from build123d import *

# Parameters (mm, degrees)
BOSS_EXTRUDE1_DEPTH = 5
SKETCH3_R           = 2.125
CUT_EXTRUDE1_DEPTH  = 10
FILLET1_R           = 10
SKETCH4_R           = 2.65
CUT_EXTRUDE2_DEPTH  = 10
SKETCH5_R           = 2.125
CUT_EXTRUDE3_DEPTH  = 10


with BuildPart() as part:
    # Sketch1 → Boss-Extrude1 (new body)
    with BuildSketch(Plane.XY):
        Polygon((0, 0), (0, 110), (166.5, 110), (166.5, 35), (223.5, 35), (223.5, 110), (278.5, 110), (278.5, 35), (335.5, 35), (335.5, 110), (502, 110), (502, 0), align=None)
    extrude(amount=BOSS_EXTRUDE1_DEPTH)

    # Sketch3 → Cut-Extrude1 (cut)
    with BuildSketch(Plane.XY.offset(5)):
        with Locations((162.5, 73)):
            Circle(SKETCH3_R)
        with Locations((162.5, 62)):
            Circle(SKETCH3_R)
        with Locations(Location((227.5, 62, 0), (0, 0, 180))):
            Circle(SKETCH3_R)
        with Locations(Location((227.5, 73, 0), (0, 0, 180))):
            Circle(SKETCH3_R)
        with Locations((274.5, 73)):
            Circle(SKETCH3_R)
        with Locations((274.5, 62)):
            Circle(SKETCH3_R)
        with Locations(Location((339.5, 62, 0), (0, 0, 180))):
            Circle(SKETCH3_R)
        with Locations(Location((339.5, 73, 0), (0, 0, 180))):
            Circle(SKETCH3_R)
    extrude(amount=-CUT_EXTRUDE1_DEPTH, mode=Mode.SUBTRACT)

    # Fillet1
    fillet1_edges = [part.edges().sort_by_distance(p)[0] for p in [
        (0, 0, 2.5),
        (0, 110, 2.5),
        (502, 110, 2.5),
        (502, 0, 2.5),
    ]]
    fillet(fillet1_edges, radius=FILLET1_R)

    # Sketch4 → Cut-Extrude2 (cut)
    with BuildSketch(Plane.XY.offset(5)):
        with Locations((148.5, 20)):
            Circle(SKETCH4_R)
        with Locations(Location((353.5, 20, 0), (0, 0, 180))):
            Circle(SKETCH4_R)
    extrude(amount=-CUT_EXTRUDE2_DEPTH, mode=Mode.SUBTRACT)

    # Sketch5 → Cut-Extrude3 (cut)
    with BuildSketch(Plane.XY.offset(5)):
        with Locations((365.5, 40)):
            Circle(SKETCH5_R)
        with Locations(Location((136.5, 40, 0), (0, 0, 180))):
            Circle(SKETCH5_R)
    extrude(amount=-CUT_EXTRUDE3_DEPTH, mode=Mode.SUBTRACT)


solid = part.part
Input: part model. Units: mm. Frame: model coordinates. Coordinates: 2 decimals unless noted, no trailing zeros. Write each loop counter-clockwise with the first axis right and the second up, starting at its lowest first coordinate (ties: lowest second). Pieces come first, ordered by that corner, then holes. Notation, with made-up numbers: M -26.5,25.25 L 22.5,25.25 A27 ccw 22.5,56.25 Z; hole C -13,75.25 d1. An arc over 180 degrees is marked long. Answer as a JSON object with one key per item and string values. Group by question number.
(1) Section B-B on x = 313.5. Output: boundary loops of the cut face in (y, z), plus the area to 3 significant figures.
(2) Ray query, line 1 along Y through (x, z) = (162.5, 2.5) (3 decimals); line 2 along X through (y, z) = (92, 1.5); line 3 along Y through (x, z) = (353.5, 3.25). Return the intervals inside material, ascending. Write a range as [from, to].
(3) Mould query, pull axis Z, two halves, no side actions, for faces 1 (the face through (2.85, 3.01, 2.54)), 2 (the face through (255, 56, 0)), 3 (the face through (255, 56, 5)). Classes: pulls with the +Z half, pulls with the -Z half, needs draft (parallel to the pull), parting line crosses it, or undercut.
(4) Section A-A on z = 1.55. Give the number of separate pieces and of enclosed holes in the cut face, plus the area to 3 significant figures.
(5) Contact query for a flat-ended pin moving along its axis: P1, Ø2.5, axis at x = 339.5, y = 62, coming from the +Z side. Output: stop coordinate, or through.
Result set:
{
 "1": {"outline": "M 0,0 L 35,0 L 35,5 L 0,5 Z", "area": "175 mm2"},
 "2": {"line 1": "y = [0, 59.875], [64.125, 70.875], [75.125, 110]", "line 2": "x = [0, 166.5], [223.5, 278.5], [335.5, 502]", "line 3": "y = [0, 17.35], [22.65, 110]"},
 "3": {"face 1": "needs draft", "face 2": "pulls with the -Z half", "face 3": "pulls with the +Z half"},
 "4": {"separate pieces": "1", "enclosed holes": "12", "area": "46,400 mm2"},
 "5": {"P1": "passes through"}
}
